from build123d import *

# Parameters (mm, degrees)
SKETCH1_W                                           = 80
SKETCH1_H                                           = 80
BOSS_EXTRUDE1_DEPTH                                 = 30
SKETCH2_W                                           = 74
SKETCH2_H                                           = 74
CUT_EXTRUDE1_DEPTH                                  = 27
CUT_EXTRUDE2_DEPTH                                  = 3
SKETCH5_W                                           = 3
SKETCH5_H                                           = 3
BOSS_EXTRUDE3_DEPTH                                 = 27
SKETCH6_W                                           = 3
SKETCH6_H                                           = 3
BOSS_EXTRUDE4_DEPTH                                 = 27
CSK_FOR_M2_COUNTERSUNK_FLAT_HEAD_SCREW1_D           = 2.4
CSK_FOR_M2_COUNTERSUNK_FLAT_HEAD_SCREW1_CSINK_D     = 4.4
CSK_FOR_M2_COUNTERSUNK_FLAT_HEAD_SCREW1_CSINK_ANGLE = 90
BOSS_EXTRUDE5_DEPTH                                 = 3
SKETCH10_W                                          = 5
SKETCH10_H                                          = 5
BOSS_EXTRUDE6_DEPTH                                 = 19


with BuildPart() as part:
    # Sketch1 → Boss-Extrude1 (new body)
    with BuildSketch(Plane.XY):
        with Locations((40, 40)):
            Rectangle(SKETCH1_W, SKETCH1_H)
    extrude(amount=BOSS_EXTRUDE1_DEPTH)

    # Sketch2 → Cut-Extrude1 (cut)
    with BuildSketch(Plane.XY.offset(30)):
        with Locations((40, 40)):
            Rectangle(SKETCH2_W, SKETCH2_H)
    extrude(amount=-CUT_EXTRUDE1_DEPTH, mode=Mode.SUBTRACT)

    # Sketch3 → Cut-Extrude2 (cut)
    with BuildSketch(Plane(origin=(80, 0, 0), x_dir=(0, 0, -1), z_dir=(1, 0, 0))):
        Polygon((-3, 68), (-3, 63), (-10, 63), (-10, 68), (-10, 73), (-3, 73), align=None)
    extrude(amount=-CUT_EXTRUDE2_DEPTH, mode=Mode.SUBTRACT)

    # Sketch5 → Boss-Extrude3 (add)
    with BuildSketch(Plane.XY.offset(3)):
        with Locations((4.5, 75.5)):
            Rectangle(SKETCH5_W, SKETCH5_H)
    extrude(amount=BOSS_EXTRUDE3_DEPTH)

    # Sketch6 → Boss-Extrude4 (add)
    with BuildSketch(Plane.XY.offset(3)):
        with Locations((75.5, 4.5)):
            Rectangle(SKETCH6_W, SKETCH6_H)
    extrude(amount=BOSS_EXTRUDE4_DEPTH)

    # CSK for M2 Countersunk Flat Head Screw1 (through all)
    with Locations(Plane.XY.offset(30)):
        with Locations((3, 77), (77, 3)):
            CounterSinkHole(CSK_FOR_M2_COUNTERSUNK_FLAT_HEAD_SCREW1_D / 2, CSK_FOR_M2_COUNTERSUNK_FLAT_HEAD_SCREW1_CSINK_D / 2, counter_sink_angle=CSK_FOR_M2_COUNTERSUNK_FLAT_HEAD_SCREW1_CSINK_ANGLE)

    # Sketch9 → Boss-Extrude5 (add)
    with BuildSketch(Plane.XY.offset(3)):
        Polygon((50, 68), (50, 69), (47.538755388, 69), (47.538755388, 68), (47.538755388, 67), (50, 67), align=None)
    extrude(amount=BOSS_EXTRUDE5_DEPTH)

    # Sketch10 → Boss-Extrude6 (add)
    with BuildSketch(Plane.XY.offset(3)):
        with Locations((67.5, 56.5)):
            Rectangle(SKETCH10_W, SKETCH10_H)
    extrude(amount=BOSS_EXTRUDE6_DEPTH)


solid = part.part
Could you check a few things on this model? Use its own coordinates, in mm. A direction names the side the tool comes from. Round coordinates to 2 decimals unless told otherwise and drop trailing zeros. Write each loop counter-clockwise with the first axis right and the second up, starting at its lowest first coordinate (ties: lowest second). Pieces come first, ordered by that corner, then holes. Notation, with made-up numbers: (82, 85) -> (130, 85) arc R28 ccw to (130, 110) -> close; hole circle Ø4 at (82, 64). An arc over 180 degrees is marked (long way). Use a Markdown table: item, result.
1. If we section it at B-B (y = 71.5): List the corners of the cut face in (x, z) for me, then the cut area to 3 significant figures.
Answer key:
| item | result |
|---|---|
| outline | (0, 0) -> (80, 0) -> (80, 3) -> (3, 3) -> (3, 30) -> (0, 30) -> close; (77, 10) -> (80, 10) -> (80, 30) -> (77, 30) -> close |
| area | 381 mm^2 |
2. Which directions (+Z, -Z, +X, -X, +Y, -Y) give clear straight access to the entire face, cutting with the end or side of a thin tool? Please do faces 1 (the face through (79, 73, 7)), 2 (the face through (3.16, 78.19, 14.3)), 3 (the face through (49, 68, 6)), 4 (the face through (39, 0, 15)), 5 (the face through (67, 59, 12)).
Answer key:
| item | result |
|---|---|
| face 1 | +X |
| face 2 | +Z, -Z |
| face 3 | +Z, +X |
| face 4 | +Z, -Z, +X, -X, -Y |
| face 5 | +Z |
3. Please list where these lines run through material, in increasing order: probe 1 along X at (y, z) = (32.5, 5); probe 2 along Z at (x, y) = (58, 10.5).
Answer key:
| item | result |
|---|---|
| probe 1 | x = 0 to 3, 77 to 80 |
| probe 2 | z = 0 to 3 |
4. We'd pull the mould along X, two halves only. Please class faces 6 (the face through (67, 54, 12)), 7 (the face through (50, 68, 4)), 8 (the face through (39, 80, 15)): +X half, -X half, draft (parallel to the pull), parting line (faces both ways), or undercut.
Answer key:
| item | result |
|---|---|
| face 6 | undercut |
| face 7 | +X half |
| face 8 | draft |
5. For pin 1 Ø2 at (x, z) = (49, 24) entering from -Y; pin 2 Ø2 at (x, y) = (54, 15) entering from +Z; pin 3 Ø1.9 at (x, y) = (3, 77) entering from +Z; pin 4 Ø2 at (y, z) = (68, 4.5) entering from +X, each with a flat end and sliding along its axis, tell me the tip position at first contact or that it passes through.
Answer key:
| item | result |
|---|---|
| pin 1 | stops at y = 0 |
| pin 2 | stops at z = 3 |
| pin 3 | passes through |
| pin 4 | stops at x = 50 |
6. If we section it at A-A (z = 28): List the corners of the cut face in (x, y) for me, then the cut area to 3 significant figures.
Answer key:
| item | result |
|---|---|
| outline | (0, 0) -> (80, 0) -> (80, 80) -> (0, 80) -> close; hole circle Ø2.4 at (3, 77); hole (3, 3) -> (74, 3) -> (74, 6) -> (77, 6) -> (77, 77) -> (6, 77) -> (6, 74) -> (3, 74) -> close; hole circle Ø2.4 at (77, 3) |
| area | 933 mm^2 |
7. If we section it at C-C (x = 58): List the corners of the cut face in (y, z) for me, then the cut area to 3 significant figures.
Answer key:
| item | result |
|---|---|
| outline | (0, 0) -> (80, 0) -> (80, 30) -> (77, 30) -> (77, 3) -> (3, 3) -> (3, 30) -> (0, 30) -> close |
| area | 402 mm^2 |
